Here's the drawing with two shaded views (mm, measured from the low corner). I have some questions. A direction names the side the tool comes from. Give positions to 0.01 mm unless a question says otherwise; leave off trailing zeros. Loops run counter-clockwise (first coordinate to the right, second up) from the corner with the lowest first, then second, coordinate; pieces in that order, holes last. Notation, with made-up numbers: M 19.25,25 L 52.25,25 A20 cw 52.25,30 Z; hole C -39.5,-20.5 d10. An arc over 180 degrees is marked long. Write item = value, one per line. Start each with the question number.
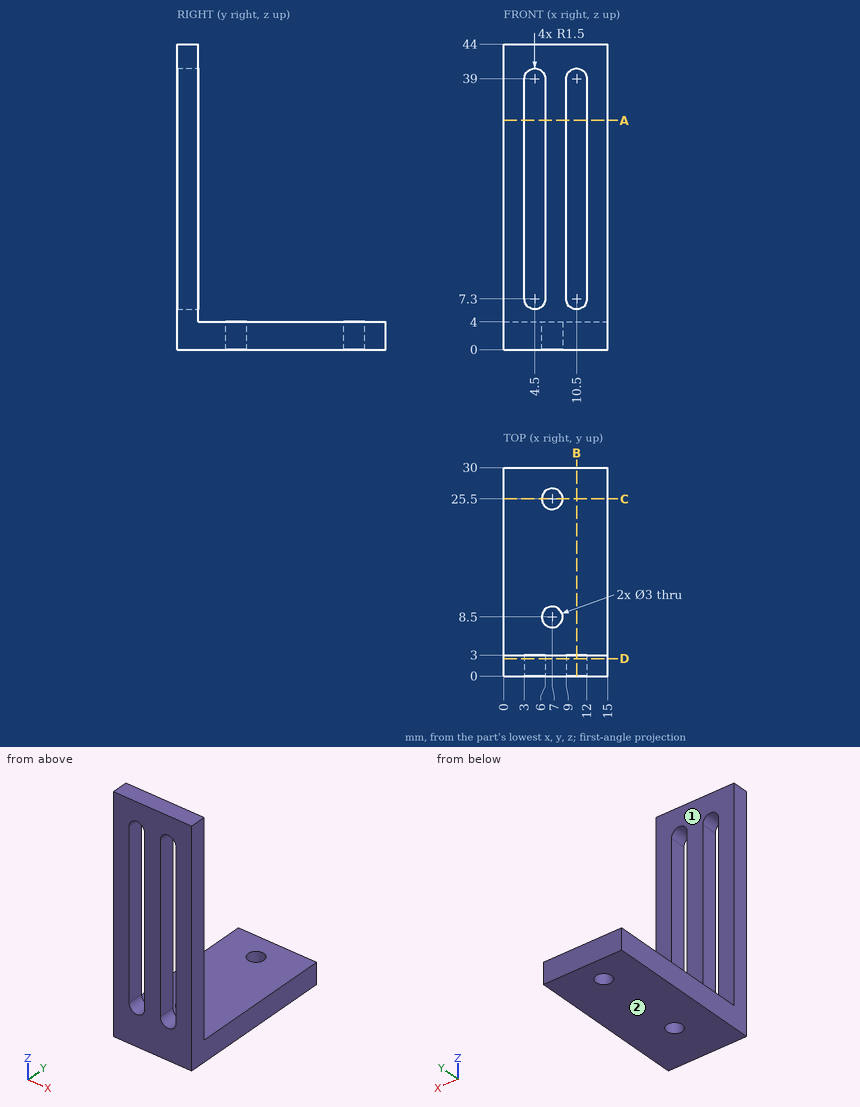
Q1. If we section it at B-B, the plane x = 10.5: List the corners of the cut face in (y, z) for me, then the cut area to 3 significant figures.
Q2. On a 3-axis mill with a long thin cutter (end or side, diameter ignored), from which of +Z, -Z, +X, -X, +Y, -Y can I reach the whole of each face in a straight line? I mean the marked faces 1 and 2. Say none if no direction works.
Q3. If we section it at C-C, the plane y = 25.5: List the corners of the cut face in (x, z) for me, then the cut area to 3 significant figures.
Q4. If I drill on line 1 along Y through (x, z) = (7, 2.6); line 2 along Z through (x, y) = (11.5, 15); line 3 along Z through (x, y) = (3.5, 1.25), over which ranges is the centre line in solid material (lowest first)?
Q5. Will these pins go through, and if not, where does the flat tip stop? pin 1 (1 mm diameter, centred on x = 7, y = 24, fed in from +Z); pin 2 (4.5 mm diameter, centred on x = 7, z = 14.5, fed in from +Y).
Q6. If we section it at D-D, the plane y = 2.5: List the corners of the cut face in (x, z) for me.
Q7. If we section it at A-A, the plane z = 33: List the corners of the cut face in (x, y) for me.
Resolved:
q1.outline = M 0,0 L 30,0 L 30,4 L 3,4 L 3,5.8 L 0,5.8 Z; M 0,40.5 L 3,40.5 L 3,44 L 0,44 Z
q1.area = 136 mm²
q2.face_1 = +Z, +X, -X, +Y
q2.face_2 = -Z, +X, -X, +Y, -Y
q3.outline = M 0,0 L 5.5,0 L 5.5,4 L 0,4 Z; M 8.5,0 L 15,0 L 15,4 L 8.5,4 Z
q3.area = 48.0 mm²
q4.line_1 = 0 to 7, 10 to 24, 27 to 30
q4.line_2 = 0 to 4
q4.line_3 = 0 to 6.18, 40.12 to 44
q5.pin_1 = 4
q5.pin_2 = 3
q6.outline = M 0,0 L 15,0 L 15,44 L 0,44 Z; hole M 3,7.3 A1.5 ccw 6,7.3 L 6,39 A1.5 ccw 3,39 Z; hole M 9,7.3 A1.5 ccw 12,7.3 L 12,39 A1.5 ccw 9,39 Z
q7.outline = M 0,0 L 3,0 L 3,3 L 0,3 Z; M 6,0 L 9,0 L 9,3 L 6,3 Z; M 12,0 L 15,0 L 15,3 L 12,3 Z
